Source: CAD feature listing. Evaluate the final solid. Frame: model axes, mm. Face numbers are marked on the shaded views. Round coordinates to 2 decimals unless told otherwise and drop trailing zeros. Loops run counter-clockwise (first coordinate to the right, second up) from the corner with the lowest first, then second, coordinate; pieces in that order, holes last. Notation, with made-up numbers: (80, 11) - (97, 11) arc R21 ccw to (97, 46) - close; hole circle Ø4 at (44, 25.5). An arc over 180 degrees is marked (long way). One line per question, with ' | ' between items. Start each with the question number.
1. Mould query, pull axis X, two halves, no side actions, for the marked faces 1 and 2. Classes: pulls with the +X half, pulls with the -X half, needs draft (parallel to the pull), parting line crosses it, or undercut.
2. Ray query, line 1 (Y direction, x = -213.5, z = -2.25); line 2 (X direction, y = -183.5, z = -18); line 3 (Z direction, x = -15.5, y = -10.5). Return the intervals inside material, ascending.
3. Cut plane A-A (z = -23.5). Return loops of the section in (x, y).
4. Pin query (flat end, axial travel): pin 1 (2 mm diameter, centred on x = -43.5, y = -403, fed in from -Z). Return the tip coordinate at first contact, or that it passes through.
5. Cut plane D-D (y = -83). Return loops of the section in (x, z).
6. Cut plane B-B (y = -414). Return loops of the section in (x, z).
7. Cut plane C-C (x = -187). Return loops of the section in (y, z).
```python
from build123d import *

# Parameters (mm, degrees)
SKETCH1_W           = 337
SKETCH1_H           = 515
SKETCH1_W_2         = 46
SKETCH1_H_2         = 20
BOSS_EXTRUDE1_DEPTH = 10
SKETCH2_W           = 46
SKETCH2_H           = 515
BOSS_EXTRUDE2_DEPTH = 20


with BuildPart() as part:
    # Sketch1 → Boss-Extrude1 (new body)
    with BuildSketch(Plane.XY):
        with Locations((-99.5, -207.5)):
            Rectangle(SKETCH1_W, SKETCH1_H)
        with Locations((-199, -415)):
            Rectangle(SKETCH1_W_2, SKETCH1_H_2, mode=Mode.SUBTRACT)
        with Locations((0, -415)):
            Rectangle(SKETCH1_W_2, SKETCH1_H_2, mode=Mode.SUBTRACT)
        with Locations((-199, 0)):
            Rectangle(SKETCH1_W_2, SKETCH1_H_2, mode=Mode.SUBTRACT)
        Rectangle(SKETCH1_W_2, SKETCH1_H_2, mode=Mode.SUBTRACT)
    extrude(amount=-BOSS_EXTRUDE1_DEPTH)

    # Sketch2 → Boss-Extrude2 (add)
    with BuildSketch(Plane(origin=(0, 0, -10), x_dir=(-1, 0, 0), z_dir=(0, 0, -1))):
        with Locations((245, -207.5)):
            Rectangle(SKETCH2_W, SKETCH2_H)
        with Locations((-46, -207.5)):
            Rectangle(SKETCH2_W, SKETCH2_H)
    extrude(amount=BOSS_EXTRUDE2_DEPTH)


solid = part.part
```
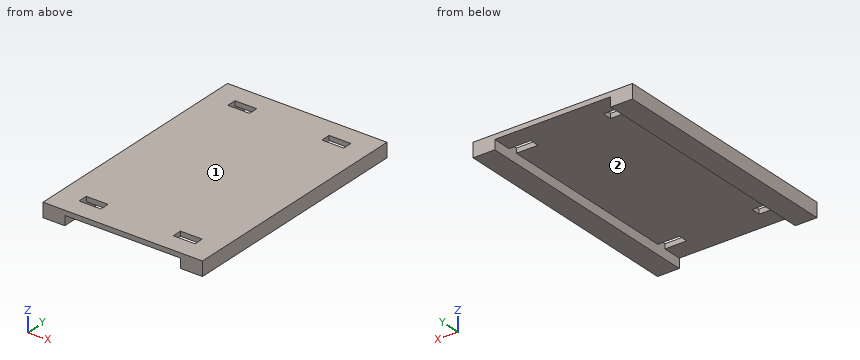
Answers follow:
1) face 1: needs draft | face 2: undercut
2) line 1: y = -465 to -425, -405 to -10, 10 to 50 | line 2: x = -268 to -222, 23 to 69 | line 3: z = -10 to 0
3) outline: (-268, -465) - (-222, -465) - (-222, 50) - (-268, 50) - close; (23, -465) - (69, -465) - (69, 50) - (23, 50) - close
4) pin 1: stops at z = -10
5) outline: (-268, -30) - (-222, -30) - (-222, -10) - (23, -10) - (23, -30) - (69, -30) - (69, 0) - (-268, 0) - close
6) outline: (-268, -30) - (-222, -30) - (-222, 0) - (-268, 0) - close; (-176, -10) - (-23, -10) - (-23, 0) - (-176, 0) - close; (23, -30) - (69, -30) - (69, 0) - (23, 0) - close
7) outline: (-465, -10) - (-425, -10) - (-425, 0) - (-465, 0) - close; (-405, -10) - (-10, -10) - (-10, 0) - (-405, 0) - close; (10, -10) - (50, -10) - (50, 0) - (10, 0) - close
